Check sheet for the drawn part. Datum: minimum x, y, z corner. Units: mm. Give positions to 0.01 mm unless a question says otherwise; leave off trailing zeros. Loops run counter-clockwise (first coordinate to the right, second up) from the corner with the lowest first, then second, coordinate; pieces in that order, holes last. Notation, with made-up numbers: M 77,68.5 L 93,68.5 A20 ccw 93,92.5 Z; hole C -4,-38 d7. An arc over 180 degrees is marked long. Write each question's results on one line, items separated by ' | '. Start each with the question number.
1. Sectioned sample at A-A on y = 1.2. Record the cut outline in (x, z) (1 decimal), and give its area (3 significant figures).
2. Sectioned sample at B-B on z = 18. Record the cut outline in (x, y).
3. Material ranges on line 1 along X through (y, z) = (1.85, 20); line 2 along Z through (x, y) = (38, 2) (1 decimal); line 3 along X through (y, z) = (0.55, 43.5) (1 decimal), recorded low to high.
4. Sectioned sample at C-C on x = 30. Record the cut outline in (y, z), and give its area (3 significant figures).
5. Go/stop test with flat-tipped pins: pin 1 (1.5 mm diameter, centred on x = 46.5, y = 3.5, fed in from -Z); pin 2 (1.5 mm diameter, centred on x = 20, y = 0.5, fed in from +Z); pin 3 (2 mm diameter, centred on x = 32, y = 1.5, fed in from +Z) (1 decimal). Record where each tip stops, or that it passes through.
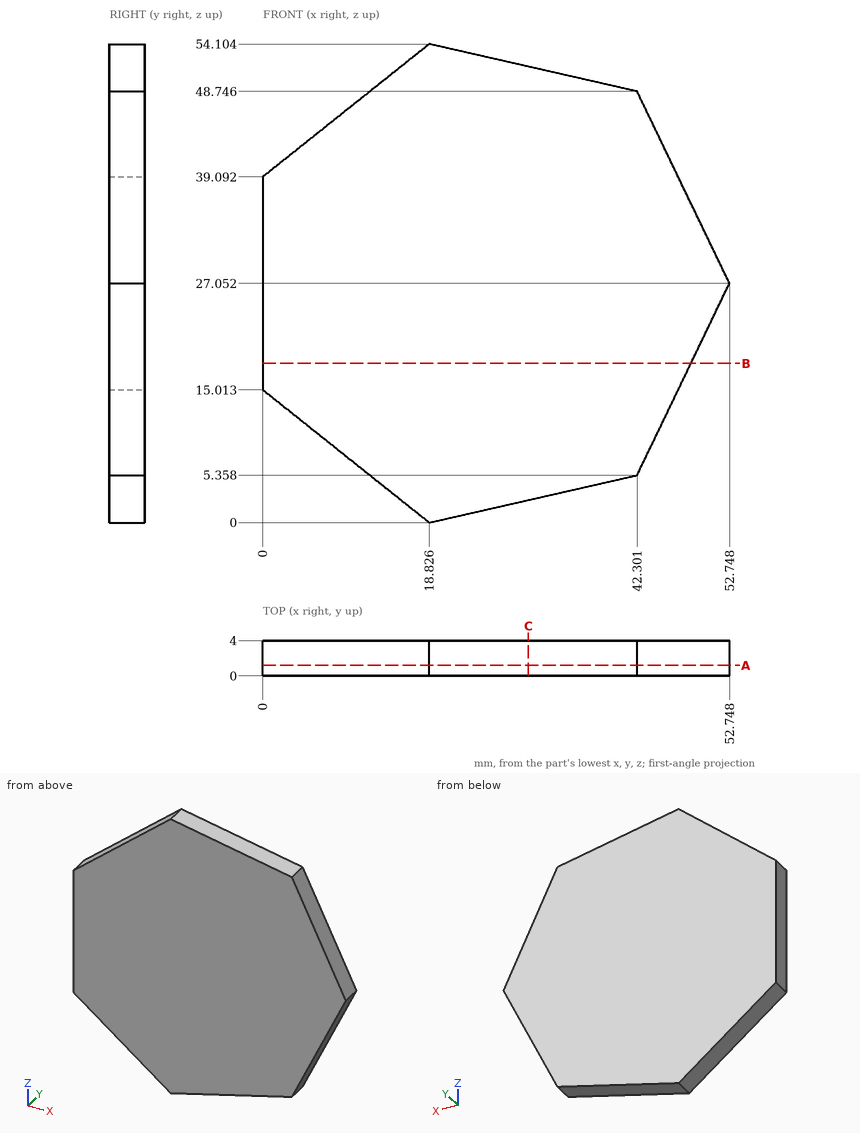
Output values:
1) outline: M 0,15 L 18.8,0 L 42.3,5.4 L 52.7,27.1 L 42.3,48.7 L 18.8,54.1 L 0,39.1 Z | area: 2,110 mm2
2) outline: M 0,0 L 48.39,0 L 48.39,4 L 0,4 Z
3) line 1: 0 to 49.35 | line 2: 4.4 to 49.7 | line 3: 5.5 to 44.8
4) outline: M 0,2.55 L 4,2.55 L 4,51.55 L 0,51.55 Z | area: 196 mm2
5) pin 1: z = 12.52 | pin 2: z = 54.01 | pin 3: z = 51.3
